Geometry: see drawing. Coordinates: mm, zero at the bounding-box minimum. A direction names the side the tool comes from. Give positions to 0.01 mm unless a question says otherwise; leave off trailing zeros. Write each loop counter-clockwise with the first axis right and the second up, starting at its lowest first coordinate (ties: lowest second). Pieces come first, ordered by that corner, then holes.
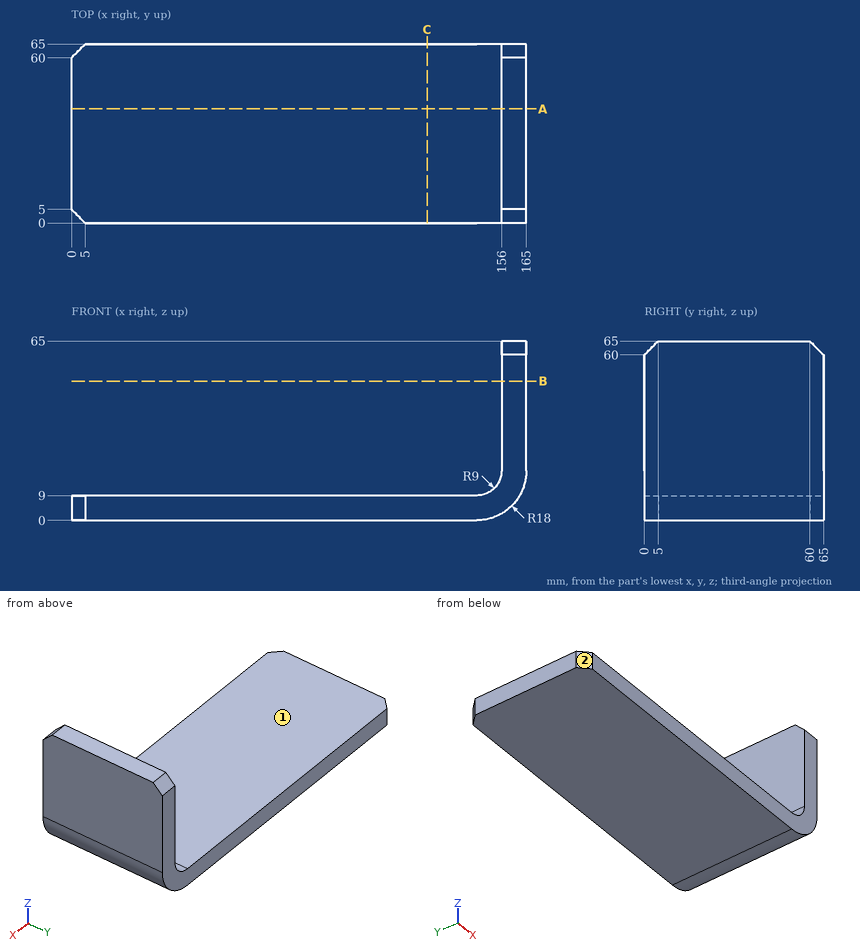
1. Pin query (flat end, axial travel): P1, Ø5, axis at y = 14, z = 49.5, coming from the -X side; P2, Ø2, axis at x = 112, y = 28, coming from the +Z side; P3, Ø12, axis at y = 41.5, z = 9, coming from the +X side. Return the tip coordinate at first contact, or that it passes through.
2. Section query B-B (z = 50.5). Return loops of the section in (x, y), plus the area to 3 significant figures.
3. Section query A-A (y = 41.5). Return loops of the section in (x, z).
4. Section query C-C (x = 129). Return loops of the section in (y, z), plus the area to 3 significant figures.
5. Access query for the marked faces 1 and 2. Directions: +Z, -Z, +X, -X, +Y, -Y. A direction counts if a zero-diameter tool reaches every point of the face in a straight line with its end or side. Return the directions, or none.
6. Line query: probe 1 along X at (y, z) = (14, 33); probe 2 along Z at (x, y) = (47.5, 13); probe 3 along X at (y, z) = (17.5, 6). Output: solid intervals per line, ascending.
The answers:
1. P1: stops at x = 156
1. P2: stops at z = 9
1. P3: stops at x = 164.75
2. outline: (156, 0) - (165, 0) - (165, 65) - (156, 65) - close
2. area: 585 mm2
3. outline: (0, 0) - (147, 0) arc R18 ccw to (165, 18) - (165, 65) - (156, 65) - (156, 18) arc R9 cw to (147, 9) - (0, 9) - close
4. outline: (0, 0) - (65, 0) - (65, 9) - (0, 9) - close
4. area: 585 mm2
5. face 1: +Z, -X, +Y, -Y
5. face 2: +Z, -Z, -X, -Y
6. probe 1: x = 156 to 165
6. probe 2: z = 0 to 9
6. probe 3: x = 0 to 160.42
